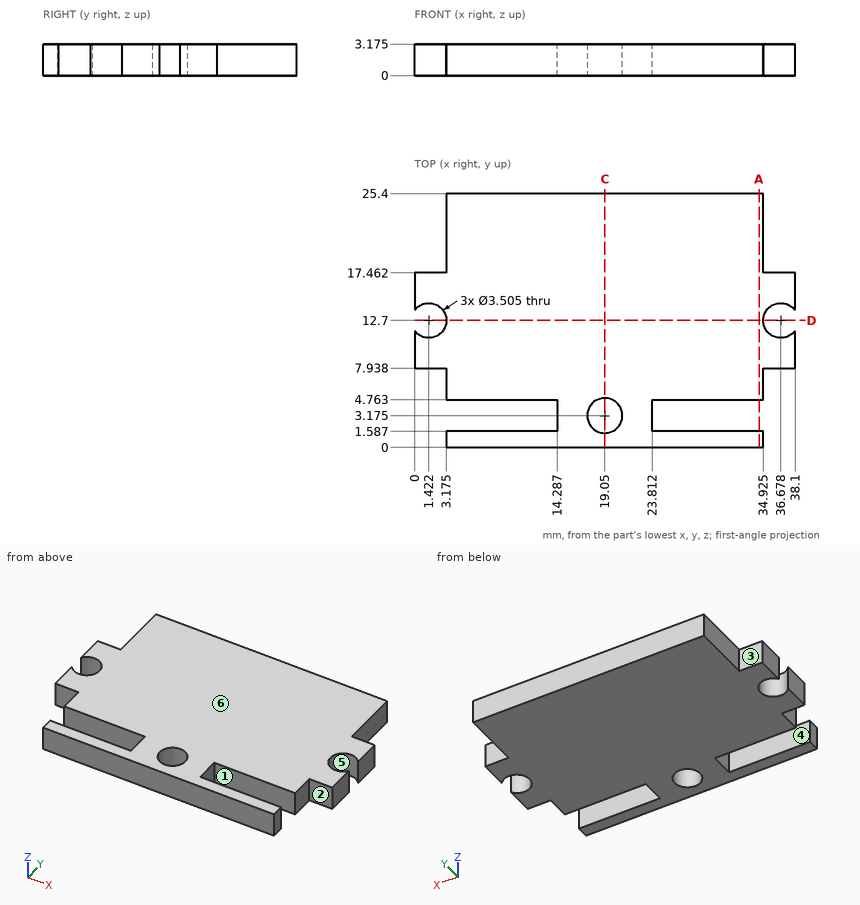
Verification items for this drawing (mm, ordinates from the low corner). A direction names the side the tool comes from. Coordinates: 2 decimals unless noted, no trailing zeros. Loops run counter-clockwise (first coordinate to the right, second up) from the corner with the lowest first, then second, coordinate; pieces in that order, holes last. Notation, with made-up numbers: (43, 42.25) - (81, 42.25) arc R18 ccw to (81, 54.25) - close; hole circle Ø7 at (46, 14). An arc over 180 degrees is marked (long way). One line per item, written item: value. Start each with the question number.
(1) Cross-section at D-D on y = 12.7. Enter the section's corners in (x, z) (1 decimal), plus the area to 3 significant figures.
(2) Material ranges on line 1 (Y direction, x = 10, z = 0.5); line 2 (X direction, y = 3.25, z = 2.6); line 3 (X direction, y = 19, z = 0.5) (1 decimal), recorded low to high. Write a range as [from, to].
(3) Depth check by flat-ended pin: P1, Ø0.8, axis at y = 0.5, z = 1, coming from the -X side (1 decimal); P2, Ø1, axis at x = 1.5, z = 1.5, coming from the -Y side; P3, Ø0.8, axis at y = 1, z = 2, coming from the +X side (1 decimal). Enter the tip coordinate at first touch or a pass-through.
(4) Cross-section at A-A on x = 34.5. Enter the section's corners in (y, z) (1 decimal).
(5) Cross-section at C-C on x = 19.05. Enter the section's corners in (y, z) (1 decimal).
(6) Mould release check, pull along X, two halves, no side actions. Record for the marked faces 5 and 6: released by +X, released by -X, zero draft, split by the parting line, or undercut.
(7) Tool access check on the marked faces 1, 2, 3 and 4. Record the directions out of +Z, -Z, +X, -X, +Y, -Y that give a thin tool (end or side, any length) a straight path to the whole face; none if there is none.
Results below:
1. outline: (3.2, 0) - (34.9, 0) - (34.9, 3.2) - (3.2, 3.2) - close
1. area: 101 mm2
2. line 1: y = [0, 1.59], [4.76, 25.4]
2. line 2: x = [14.29, 17.3], [20.8, 23.81]
2. line 3: x = [3.2, 34.9]
3. P1: stops at x = 3.2
3. P2: stops at y = 7.94
3. P3: stops at x = 34.9
4. outline: (0, 0) - (1.6, 0) - (1.6, 3.2) - (0, 3.2) - close; (4.8, 0) - (25.4, 0) - (25.4, 3.2) - (4.8, 3.2) - close
5. outline: (0, 0) - (1.4, 0) - (1.4, 3.2) - (0, 3.2) - close; (4.9, 0) - (25.4, 0) - (25.4, 3.2) - (4.9, 3.2) - close
6. face 5: undercut
6. face 6: zero draft
7. face 1: +Z, -Z, +X
7. face 2: +Z, -Z, +X, -Y
7. face 3: +Z, -Z, -X, +Y
7. face 4: +Z, -Z, -X
